For this review, take the finished solid that the model builds, in its own axes (mm). Face numbers are marked on the shaded views. A direction names the side the tool comes from. Give positions to 0.01 mm unless a question says otherwise; leave off trailing zeros. Order: outer loops, then holes, each group sorted by start corner. A loop starts at its lowest first (then second) coordinate and runs counter-clockwise, first axis right, second up. Notation, with made-up numbers: M 56,77.5 L 63,77.5 A20 cw 63,104.5 Z; hole C -28.5,59.25 d10. An arc over 180 degrees is marked long. Answer as CSV lines item,"result". Start each with the question number.
1. Clearance check with flat-ended pins moving along their axes: P1, Ø5, axis at y = 2.5, z = 6.5, coming from the -X side; P2, Ø3, axis at y = 8.5, z = 7.5, coming from the -X side; P3, Ø7, axis at x = 1, z = 1.5, coming from the -Y side. State where each tip first meets the part, or that it passes through.
2. For line 1 along X through (y, z) = (4, 13.5); line 2 along X through (y, z) = (3.5, -11); line 3 along X through (y, z) = (14.25, -7.25), list the stretches that pass through material, from the lowest coordinate up.
3. We need section B-B, the plane y = 7.5. Give the boundary of the cut face in (x, z), and give its area (3 significant figures).
4. We need section D-D, the plane y = 13.5. Give the boundary of the cut face in (x, z), and give its area (3 significant figures).
5. Machinability: for the marked faces 1, 2 and 3, which of the approach directions +Z, -Z, +X, -X, +Y, -Y give a long, thin tool a straight path to every point of the face, cutting with its end or side? Answer none if there is none.
6. We need section C-C, the plane y = 10.5. Give the boundary of the cut face in (x, z), and give its area (3 significant figures).
7. We need section A-A, the plane x = 0. State how many separate pieces and enclosed holes the cut face has, and give its area (3 significant figures).
8. Mouldability with a two-part tool opening along Z and no side actions: class the marked faces 4, 5 and 6 as pulls with the +Z half, pulls with the -Z half, needs draft (parallel to the pull), parting line crosses it, or undercut.
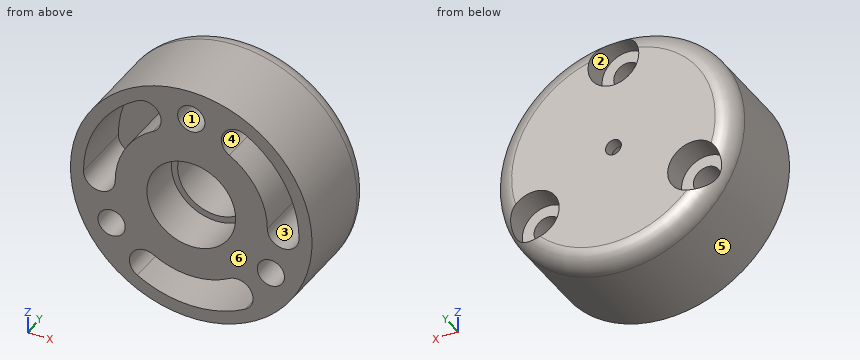
from build123d import *

# Parameters (mm, degrees)
SKETCH1_R                      = 19.05
BOSS_EXTRUDE1_DEPTH            = 15.875
SKETCH2_R                      = 7
CUT_EXTRUDE1_DEPTH             = 7
SKETCH3_R                      = 6
CUT_EXTRUDE2_DEPTH             = 7
M3X0_5_TAPPED_HOLE1_D          = 2.5
CBORE_FOR_M4_SHCS1_D           = 4.3
CBORE_FOR_M4_SHCS1_CBORE_D     = 8
CBORE_FOR_M4_SHCS1_CBORE_DEPTH = 4
CIRPATTERN1_COUNT              = 3
FILLET1_R                      = 3
CUT_EXTRUDE3_DEPTH             = 10
CIRPATTERN2_COUNT              = 3


with BuildPart() as part:
    # Sketch1 → Boss-Extrude1 (new body)
    with BuildSketch(Plane(origin=(0, 0, 0), x_dir=(1, 0, 0), z_dir=(0, 1, 0))):
        with Locations(Location((0, 0, 0), (0, 0, 270))):
            Circle(SKETCH1_R)
    extrude(amount=BOSS_EXTRUDE1_DEPTH)

    # Sketch2 → Cut-Extrude1 (cut)
    with BuildSketch(Plane.XZ):
        with Locations(Location((0, 0, 0), (0, 0, 270))):
            Circle(SKETCH2_R)
    extrude(amount=-CUT_EXTRUDE1_DEPTH, mode=Mode.SUBTRACT)

    # Sketch3 → Cut-Extrude2 (cut)
    with BuildSketch(Plane.XZ.offset(-7)):
        with Locations(Location((0, 0, 0), (0, 0, 270))):
            Circle(SKETCH3_R)
    extrude(amount=-CUT_EXTRUDE2_DEPTH, mode=Mode.SUBTRACT)

    # M3x0.5 Tapped Hole1 (through all)
    with Locations(Plane.XZ.offset(-14)):
        with Locations((0, 0)):
            Hole(M3X0_5_TAPPED_HOLE1_D / 2)

    # CBORE for M4 SHCS1 (through all)
    with Locations(Plane(origin=(0, 15.875, 0), x_dir=(-1, 0, 0), z_dir=(0, 1, 0))):
        with Locations((0, 14.5)):
            cbore_for_m4_shcs1 = CounterBoreHole(CBORE_FOR_M4_SHCS1_D / 2, CBORE_FOR_M4_SHCS1_CBORE_D / 2, CBORE_FOR_M4_SHCS1_CBORE_DEPTH)

    # CirPattern1: CBORE for M4 SHCS1 ×3 about axis
    cirpattern1_axis = Axis((0, 0, 0), (0, 1, 0))
    for i in range(1, CIRPATTERN1_COUNT):
        add(cbore_for_m4_shcs1.rotate(cirpattern1_axis, i * 360 / CIRPATTERN1_COUNT), mode=Mode.SUBTRACT)

    # Fillet1
    # the kernel refuses this fillet: 3 mm, written as the material it takes off along each edge
    with BuildSketch(Plane(origin=(0, 15.875, 0), x_dir=(0, 0, 1), z_dir=(-1, 0, 0))) as fillet1_piece_1:
        with BuildLine():
            CenterArc((19.05 - FILLET1_R, -FILLET1_R), FILLET1_R, 0, 90)
            Line((19.05 - FILLET1_R, 0), (19.05, 0))
            Line((19.05, 0), (19.05, -FILLET1_R))
        make_face()
    revolve(axis=Axis((0, 15.875, 0), (0, 1, 0)), mode=Mode.SUBTRACT)

    # Sketch9 → Cut-Extrude3 (cut)
    with BuildSketch(Plane.XZ):
        with BuildLine():
            ThreePointArc((-6, 10.392304845), (-5.084936491, 13.807368355), (-8.5, 14.722431864))
            ThreePointArc((-8.5, 14.722431864), (-14.722431864, 8.5), (-17, 0))
            ThreePointArc((-17, 0), (-14.5, -2.5), (-12, 0))
            ThreePointArc((-12, 0), (-10.392304845, 6), (-6, 10.392304845))
        make_face()
    cut_extrude3 = extrude(amount=-CUT_EXTRUDE3_DEPTH, mode=Mode.SUBTRACT)

    # CirPattern2: Cut-Extrude3 ×3 about axis
    cirpattern2_axis = Axis((0, 0, 0), (0, 1, 0))
    for i in range(1, CIRPATTERN2_COUNT):
        add(cut_extrude3.rotate(cirpattern2_axis, i * 360 / CIRPATTERN2_COUNT), mode=Mode.SUBTRACT)


solid = part.part
Result set:
1,P1,"x = -18.63"
1,P2,"x = -18.08"
1,P3,"y = 14"
2,line 1,"-13.44 to -10.33, -4.93 to -1.9, 1.9 to 4.93, 10.33 to 13.44"
2,line 2,"-15.55 to -9.21, -4.8 to 4.8, 9.21 to 15.55"
2,line 3,"-17.26 to -16.56, -8.56 to 8.56, 16.56 to 17.26"
3,outline,"C 0,0 d38.1; hole M -17,0 A2.5 ccw -12,0 A12 cw -6,10.39 A2.5 ccw -8.5,14.72 A17 ccw Z; hole C -12.56,-7.25 d4.3; hole M -8.5,-14.72 A17 ccw 8.5,-14.72 A2.5 ccw 6,-10.39 A12 cw -6,-10.39 A2.5 ccw Z; hole C 0,0 d12; hole C 0,14.5 d4.3; hole M 6,10.39 A12 cw 12,0 A2.5 ccw 17,0 A17 ccw 8.5,14.72 A2.5 ccw Z; hole C 12.56,-7.25 d4.3"
3,area,"697 mm2"
4,outline,"C 0,0 d37.97; hole C -12.56,-7.25 d8; hole C 0,0 d12; hole C 0,14.5 d8; hole C 12.56,-7.25 d8"
4,area,"868 mm2"
5,face 1,"+Y, -Y"
5,face 2,"+Y"
5,face 3,"-Y"
6,outline,"C 0,0 d38.1; hole C -12.56,-7.25 d4.3; hole C 0,0 d12; hole C 0,14.5 d4.3; hole C 12.56,-7.25 d4.3"
6,area,"983 mm2"
7,separate pieces,"3"
7,enclosed holes,"0"
7,area,"282 mm2"
8,face 4,"undercut"
8,face 5,"parting line crosses it"
8,face 6,"needs draft"
